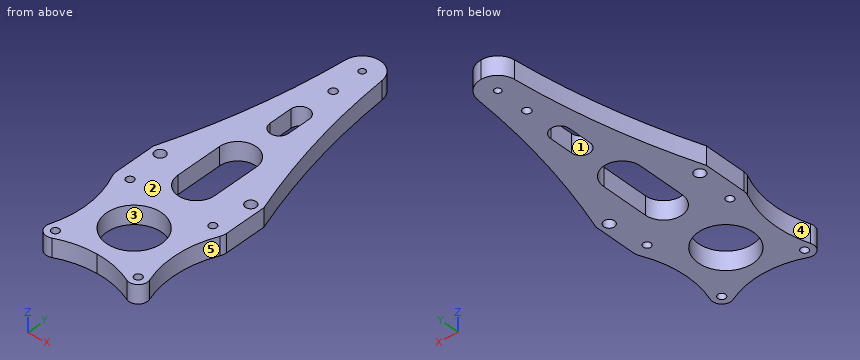
```python
from build123d import *

# Parameters (mm, degrees)
ESQUISSE1_R             = 4.1
ESQUISSE1_R_2           = 5.75
BOSS_EXTRU_1_DEPTH      = 20
ESQUISSE2_R             = 30
ENL_V_MAT_EXTRU_1_DEPTH = 20
ENL_V_MAT_EXTRU_2_DEPTH = 20
ENL_V_MAT_EXTRU_3_DEPTH = 20
ESQUISSE5_R             = 4.25
ENL_V_MAT_EXTRU_4_DEPTH = 20
TROU_TARAUD_M8X1_01_D   = 7


with BuildPart() as part:
    # Esquisse1 → Boss.-Extru.1 (new body)
    with BuildSketch(Plane.XY):
        with BuildLine():
            Line((0, 0), (0, -340))
            ThreePointArc((0, -340), (-20.879556565, -342.291995457), (-40.764705882, -349.058823529))
            ThreePointArc((-40.764705882, -349.058823529), (-51.70200076, -347.421804754), (-54.442463892, -336.707603359))
            ThreePointArc((-54.442463892, -336.707603359), (-48.641150346, -296.132285263), (-58.581232197, -256.367898556))
            ThreePointArc((-58.581232197, -256.367898556), (-59.641012311, -253.262017554), (-60, -250))
            Line((-60, -250), (-60, -205))
            ThreePointArc((-60, -205), (-34.0967157, -112.901065178), (-19.926246382, -18.283985684))
            ThreePointArc((-19.926246382, -18.283985684), (-13.521828901, -5.263645527), (0, 0))
        make_face()
        with Locations((-45, -340)):
            Circle(ESQUISSE1_R, mode=Mode.SUBTRACT)
        with Locations((-45, -250)):
            Circle(ESQUISSE1_R, mode=Mode.SUBTRACT)
        with Locations((-49.25, -209)):
            Circle(ESQUISSE1_R_2, mode=Mode.SUBTRACT)
    boss_extru_1 = extrude(amount=BOSS_EXTRU_1_DEPTH)

    # Symétrie1: Boss.-Extru.1 across plane
    add(boss_extru_1.mirror(Plane(origin=(0, 0, 20), x_dir=(0, 0, 1), z_dir=(-1, 0, 0))))

    # Esquisse2 → Enlèv. mat.-Extru.1 (cut)
    with BuildSketch(Plane.XY.offset(20)):
        with Locations((0, -295)):
            Circle(ESQUISSE2_R)
    extrude(amount=-ENL_V_MAT_EXTRU_1_DEPTH, mode=Mode.SUBTRACT)

    # Esquisse3 → Enlèv. mat.-Extru.2 (cut)
    with BuildSketch(Plane.XY.offset(20)):
        with BuildLine():
            Line((-20, -220), (-20, -170))
            ThreePointArc((-20, -170), (0, -150), (20, -170))
            Line((20, -170), (20, -220))
            ThreePointArc((20, -220), (0, -240), (-20, -220))
        make_face()
    extrude(amount=-ENL_V_MAT_EXTRU_2_DEPTH, mode=Mode.SUBTRACT)

    # Esquisse4 → Enlèv. mat.-Extru.3 (cut)
    with BuildSketch(Plane.XY.offset(20)):
        with BuildLine():
            Line((-10, -120), (-10, -95))
            ThreePointArc((-10, -95), (0, -85), (10, -95))
            Line((10, -95), (10, -120))
            ThreePointArc((10, -120), (0, -130), (-10, -120))
        make_face()
    extrude(amount=-ENL_V_MAT_EXTRU_3_DEPTH, mode=Mode.SUBTRACT)

    # Esquisse5 → Enlèv. mat.-Extru.4 (cut)
    with BuildSketch(Plane.XY.offset(20)):
        with Locations((0, -55)):
            Circle(ESQUISSE5_R)
    extrude(amount=-ENL_V_MAT_EXTRU_4_DEPTH, mode=Mode.SUBTRACT)

    # Trou taraudé M8x1.01 (through all)
    with Locations(Plane.XY.offset(20)):
        with Locations((0, -20)):
            Hole(TROU_TARAUD_M8X1_01_D / 2)


solid = part.part
```
Can you work these out from the model? Positions are in its coordinate system, mm. Face numbers are marked on the shaded views. A direction names the side the tool comes from. Coordinates: 2 decimals unless noted, no trailing zeros. Write each loop counter-clockwise with the first axis right and the second up, starting at its lowest first coordinate (ties: lowest second). Pieces come first, ordered by that corner, then holes. Notation, with made-up numbers: M -5.5,78.25 L 14.5,78.25 A14 ccw 14.5,89.25 Z; hole C 60,8 d4. An arc over 180 degrees is marked long. Answer as CSV lines item,"result".
Item 1: I'm going to push flat-ended pins straight in: P1, Ø1.5, axis at x = 13, z = 15.5, coming from the -Y side; P2, Ø1.5, axis at x = 20.5, z = 6, coming from the -Y side; P3, Ø6, axis at y = -196, z = 8.5, coming from the -X side. Where does each tip first touch, or does it pass through?
Geometry results:
P1,"stops at y = -340.99"
P2,"stops at y = -342.38"
P3,"stops at x = -57.93"
Item 2: Imagine slicing it at B-B on x = -13.5. List the corners of the cut face in (y, z) for me, plus the area to 3 significant figures.
Geometry results:
outline,"M -340.95,0 L -321.79,0 L -321.79,20 L -340.95,20 Z; M -268.21,0 L -234.76,0 L -234.76,20 L -268.21,20 Z; M -155.24,0 L -5.24,0 L -5.24,20 L -155.24,20 Z"
area,"4,050 mm2"
Item 3: On a 3-axis mill with a long thin cutter (end or side, diameter ignored), from which of +Z, -Z, +X, -X, +Y, -Y can I reach the whole of each face in a straight line? I mean the marked faces 1 and 2. Say none if no direction works.
Geometry results:
face 1,"+Z, -Z"
face 2,"+Z, +X, -X, +Y, -Y"
Item 4: Imagine slicing it at C-C on z = 10.25. State how many separate pieces and enclosed holes the cut face has, plus the area to 3 significant figures.
Geometry results:
separate pieces,"1"
enclosed holes,"11"
area,"21,800 mm2"
Item 5: Imagine slicing it at D-D on y = -162. List the corners of the cut face in (x, z) for me.
Geometry results:
outline,"M -46.35,0 L -18.33,0 L -18.33,20 L -46.35,20 Z; M 18.33,0 L 46.35,0 L 46.35,20 L 18.33,20 Z"
Item 6: Imagine slicing it at A-A on y = -198.5. List the corners of the cut face in (x, z) for me.
Geometry results:
outline,"M -57.76,0 L -20,0 L -20,20 L -57.76,20 Z; M 20,0 L 57.76,0 L 57.76,20 L 20,20 Z"
Item 7: Please list where these lines run through material, in increasing order: line 1 along X through (y, z) = (-208.5, 12); line 2 along X through (y, z) = (-250.5, 13.75); line 3 along Y through (x, z) = (0, 7.5).
Geometry results:
line 1,"x = -60 to -54.98, -43.52 to -20, 20 to 43.52, 54.98 to 60"
line 2,"x = -59.99 to -49.07, -40.93 to 40.93, 49.07 to 59.99"
line 3,"y = -340 to -325, -265 to -240, -150 to -130, -85 to -59.25, -50.75 to -23.5, -16.5 to 0"
Item 8: We'd pull the mould along X, two halves only. Please class the marked faces 3, 4 and 5: +X half, -X half, draft (parallel to the pull), parting line (faces both ways), or undercut.
Geometry results:
face 3,"undercut"
face 4,"-X half"
face 5,"+X half"
